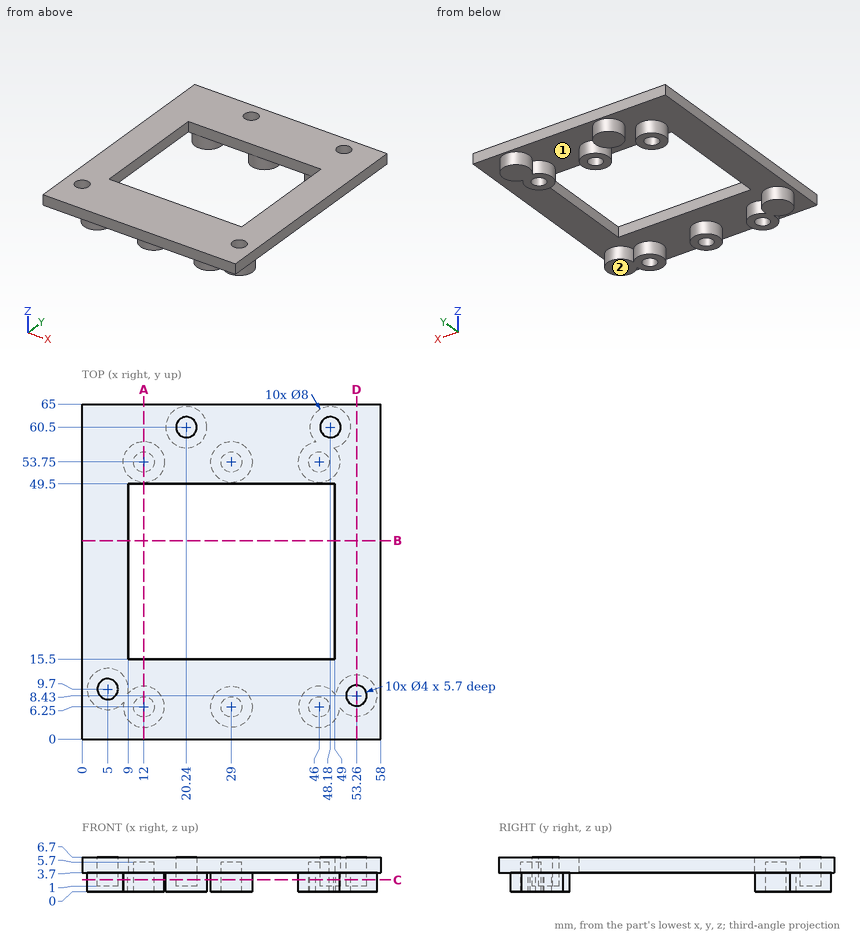
Check sheet for the drawn part. Datum: minimum x, y, z corner. Units: mm. Round coordinates to 2 decimals unless told otherwise and drop trailing zeros. Write each loop counter-clockwise with the first axis right and the second up, starting at its lowest first coordinate (ties: lowest second). Pieces come first, ordered by that corner, then holes. Notation, with made-up numbers: (23.25, 51) - (41.25, 51) arc R20 ccw to (41.25, 87) - close; hole circle Ø9 at (10.25, -16.5). An arc over 180 degrees is marked (long way). Write each question's results on one line, items separated by ' | '.
(1) Sectioned sample at B-B, the plane y = 38.5. Enter the section's corners in (x, z), plus the area to 3 significant figures.
Computed:
outline: (0, 3.7) - (9, 3.7) - (9, 6.7) - (0, 6.7) - close; (49, 3.7) - (58, 3.7) - (58, 6.7) - (49, 6.7) - close | area: 54.0 mm^2
(2) Depth check by flat-ended pin: pin 1 Ø3 at (x, y) = (48.18, 60.5) entering from +Z; pin 2 Ø2.5 at (x, y) = (29, 53.75) entering from -Z; pin 3 Ø3 at (y, z) = (43.5, 3.5) entering from +X; pin 4 Ø17.5 at (x, y) = (21, 39) entering from -Z. Enter the tip coordinate at first touch or a pass-through.
Computed:
pin 1: stops at z = 1 | pin 2: stops at z = 5.7 | pin 3: stops at x = 58 | pin 4: passes through
(3) Sectioned sample at A-A, the plane x = 12. Enter the section's corners in (y, z).
Computed:
outline: (0, 3.7) - (2.25, 3.7) - (2.25, 0) - (4.25, 0) - (4.25, 5.7) - (8.25, 5.7) - (8.25, 0) - (10.25, 0) - (10.25, 3.7) - (15.5, 3.7) - (15.5, 6.7) - (0, 6.7) - close; (49.5, 3.7) - (49.75, 3.7) - (49.75, 0) - (51.75, 0) - (51.75, 5.7) - (55.75, 5.7) - (55.75, 0) - (57.75, 0) - (57.75, 3.7) - (65, 3.7) - (65, 6.7) - (49.5, 6.7) - close
(4) Draft check along X on the marked faces 1 and 2. Enter one of: pulls with the +X half, pulls with the -X half, needs draft (parallel to the pull), parting line crosses it, or undercut.
Computed:
face 1: undercut | face 2: needs draft
(5) Sectioned sample at C-C, the plane z = 2.25. Count the separate pieces of the cut face and the enclosed holes in it, plus the area to 3 significant figures.
Computed:
separate pieces: 7 | enclosed holes: 10 | area: 374 mm^2
(6) Sectioned sample at D-D, the plane x = 53.26. Enter the section's corners in (y, z).
Computed:
outline: (0, 3.7) - (4.43, 3.7) - (4.43, 0) - (12.43, 0) - (12.43, 3.7) - (65, 3.7) - (65, 6.7) - (10.43, 6.7) - (10.43, 1) - (6.43, 1) - (6.43, 6.7) - (0, 6.7) - close
(7) Thickness scan on probe 1 along X at (y, z) = (53.75, 3.2); probe 2 along X at (y, z) = (6.25, 4); probe 3 along Y at (x, z) = (29, 1.8). Record the ranges inside material, lowest first. Write a range as from..to.
Computed:
probe 1: x = 8..10, 14..16, 25..27, 31..33, 42..44, 48..50 | probe 2: x = 0..10, 14..27, 31..44, 48..58 | probe 3: y = 2.25..4.25, 8.25..10.25, 49.75..51.75, 55.75..57.75
